Autodesk Inventor part; units mm, degrees
ref_plane "YZ Plane" through (0, 0, 0) normal (1, 0, 0) x (0, 1, 0)
ref_plane "XZ Plane" through (0, 0, 0) normal (0, 1, 0) x (-1, 0, 0)
ref_plane "XY Plane" through (0, 0, 0) normal (0, 0, 1) x (1, 0, 0)
sketch "Sketch1" plane through (0, 0, 0) normal (0, 1, 0) x (-1, 0, 0)
  circle A0 centre (0, 0) radius 1.5
  circle A1 centre (25, 2) radius 1.5
  line L0 (30, 8) -> (-14.9, 8)
  line L1 (-14.9, 8) -> (-14.9, -23)
  line L2 (-14.9, -23) -> (30, -23)
  line L3 (30, -23) -> (30, 8)
  line L4 (-14.9, -8) -> (30, -8) construction
  circle A2 centre (-9.9, 0) radius 1.5
  line L5 (25, -8) -> (20, -8)
  line L6 (20, -8) -> (20, -18)
  line L7 (20, -18) -> (25, -18)
  line L8 (25, -18) -> (25, -8)
  line L9 (20, -8) -> (20, -18)
  line L10 (20, -18) -> (15, -18)
  line L11 (15, -18) -> (15, -8)
  line L12 (15, -8) -> (20, -8)
  line L13 (15, -8) -> (15, -18)
  line L14 (15, -18) -> (10, -18)
  line L15 (10, -18) -> (10, -8)
  line L16 (10, -8) -> (15, -8)
  line L17 (-4.2, -23) -> (-14.9, -23)
  line L18 (-14.9, -23) -> (-14.9, -8)
  line L19 (-9.2, -8) -> (-9.2, -18)
  line L20 (-9.2, -18) -> (-4.2, -18)
  line L21 (-4.2, -18) -> (-4.2, -8)
  line L22 (-4.2, -8) -> (-9.2, -8)
  dimension "d0" = 3
  dimension "d1" = 3
  dimension "d3" = 25
  dimension "d4" = 2
  dimension "d5" = 8
  dimension "d6" = 6
  dimension "d7" = 5
  dimension "d9" = 3
  dimension "d10" = 9.9
  dimension "d11" = 5
  dimension "d12" = 10
  dimension "d13" = 5
  dimension "d14" = 5
  dimension "d15" = 5
  dimension "d16" = 5
  dimension "d37" = 5
  dimension "d38" = 14.2
  dimension "d39" = 5
extrude "Extrusion1" add sketch "Sketch1" along normal blind 14 contours L3 L2 L1 L0 | L6 L10 L11 L12
fillet "Fillet1" radius 2 4 edges at (-30, 7, 8) (-30, 7, -23) (14.9, 7, 8) (14.9, 7, -23)
sketch "Sketch2" plane through (-30, 0, -21) normal (-1, 0, 0) x (0, 0, 1)
  line L0 (3, 0) -> (13, 0)
  line L1 (13, 0) -> (13, 14)
  line L2 (3, 14) -> (13, 14)
  line L3 (3, 0) -> (3, 14)
  circle A0 centre (8, 11) radius 1.55
  circle A1 centre (8, 3) radius 1.55
  line L4 (3, 0) -> (3, 14)
  point P0 (21, 0)
  dimension "d21" = 3.1
  dimension "d22" = 3.1
  dimension "d23" = 3
  dimension "d24" = 3
  dimension "d35" = 5
  dimension "d36" = 5
extrude "Extrusion2" cut sketch "Sketch2" against normal blind 50 contours A0 | A1
thicken "Thicken1" operation add thickness 0.1 both sides no extend neighbours yes toward (1, 0, 0) faces at (-20, 8.0932, -9.2092) (-21.6667, 4.6667, -8) (-25, 8.0932, -9.2092) (-23.3333, 4.6667, -18)
thicken "Thicken2" operation add thickness 0.1 both sides no extend neighbours yes toward (0, 0, 1) faces at (-11.6667, 4.6667, -8) (-15, 8.0932, -9.2092) (-13.3333, 4.6667, -18) (-10, 5.9068, -16.7908)
thicken "Thicken3" operation add thickness 0.1 both sides no extend neighbours yes toward (-1, 0, 0) faces at (4.2, 8.0932, -16.7908) (5.8667, 4.6667, -18) (9.2, 5.9068, -16.7908) (7.5333, 4.6667, -8)
properties part number "Bar_connection_block"
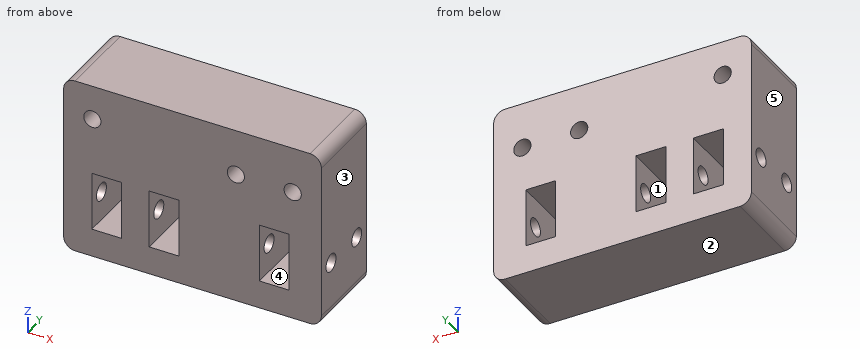
Read the model definition and answer for the solid it produces. Units are mm, in the model's axes. Face numbers are marked on the shaded views. A direction names the side the tool comes from. Coordinates: 2 decimals unless noted, no trailing zeros. Order: outer loops, then holes, each group sorted by start corner. A loop starts at its lowest first (then second) coordinate and runs counter-clockwise, first axis right, second up. Notation, with made-up numbers: M -32,86 L 21,86 A34 ccw 21,117 Z; hole C 7,86.25 d2. An arc over 180 degrees is marked long. Put each result on its own line as item: value. Start each with the question number.
Item 1: For the marked faces 4 and 5, determine the directions among +Z, -Z, +X, -X, +Y, -Y from which every point of the face is accessible in a straight line to the end or side of a thin tool.
Item 2: Section C-C, the plane x = 9.9 is taken. Determine the outline of the cut face in (y, z).
Item 3: Section A-A, the plane z = 2 is taken. Determine the outline of the cut face in (x, y), plus the area to 3 significant figures.
Item 4: Section B-B, the plane x = -11.5 is taken. Determine the outline of the cut face in (y, z), plus the area to 3 significant figures.
Item 5: Consider probe 1 along X at (y, z) = (10.75, -15.5); probe 2 along Y at (x, z) = (-6, -13); probe 3 along Z at (x, y) = (-25, 4). Determine where each line is inside the solid, lowest interval first. Write a range as [from, to].
Item 6: Section D-D, the plane y = 7.5 is taken. Determine the outline of the cut face in (x, z), plus the area to 3 significant figures.
Item 7: The mould has two halves that part along Z. Classify the marked faces 1, 2 and 3: +Z half, -Z half, draft (parallel to the pull), parting line (faces both ways), or undercut.
Computed:
1. face 4: +Y, -Y
1. face 5: +Z, -Z, -X, +Y, -Y
2. outline: M 0,-23 L 14,-23 L 14,-1.5 L 0,-1.5 Z; M 0,1.5 L 14,1.5 L 14,8 L 0,8 Z; hole C 3,-13 d3.1; hole C 11,-13 d3.1
3. outline: M -30,0 L -26.5,0 L -26.5,14 L -30,14 Z; M -23.5,0 L 14.9,0 L 14.9,14 L -23.5,14 Z
3. area: 587 mm2
4. outline: M 0,-23 L 14,-23 L 14,-18.1 L 0,-18.1 Z; M 0,-7.9 L 14,-7.9 L 14,8 L 0,8 Z
4. area: 291 mm2
5. probe 1: x = [-30, -25.1], [-19.9, -15.1], [-9.9, 4.1], [9.3, 14.9]
5. probe 2: y = [0, 1.45], [4.55, 9.45], [12.55, 14]
5. probe 3: z = [-23, -18.1], [-7.9, 0.5], [3.5, 8]
6. outline: M -30,-21 A2 ccw -28,-23 L 12.9,-23 A2 ccw 14.9,-21 L 14.9,6 A2 ccw 12.9,8 L -28,8 A2 ccw -30,6 Z; hole C -25,2 d3; hole M -25.1,-18.1 L -19.9,-18.1 L -19.9,-7.9 L -25.1,-7.9 Z; hole M -15.1,-18.1 L -9.9,-18.1 L -9.9,-7.9 L -15.1,-7.9 Z; hole C 0,0 d3; hole M 4.1,-18.1 L 9.3,-18.1 L 9.3,-7.9 L 4.1,-7.9 Z; hole C 9.9,0 d3
6. area: 1,210 mm2
7. face 1: undercut
7. face 2: -Z half
7. face 3: draft
